Part model, mm, in its own coordinate system. A direction names the side the tool comes from. Round coordinates to 2 decimals unless told otherwise and drop trailing zeros. Loops run counter-clockwise (first coordinate to the right, second up) from the corner with the lowest first, then second, coordinate; pieces in that order, holes last.
1) Band-saw the part on C-C, the plane x = 53.5. Write the cut outline in (y, z), then the cut area to 3 significant figures.
2) Band-saw the part on D-D, the plane y = 48. Write the cut outline in (x, z).
3) 3-axis set-ups, long thin cutter, end or side, ignore diameter. For faces 1 (the flat face through (37, 38, 0)), 2 (the flat face through (37, 6.35, -42)): which of +Z, -Z, +X, -X, +Y, -Y reach the whole face in a straight line?
4) Band-saw the part on B-B, the plane x = 37.5. Write the cut outline in (y, z), then the cut area to 3 significant figures.
5) Band-saw the part on A-A, the plane z = -63.5. Write the cut outline in (x, y) (3 decimals), then the cut area to 3 significant figures.
6) Mould opens along Z. For faces 3 (the cylindrical face through (13.65, 3.13, -66.53)), 4 (the cylindrical face through (68.03, 23.45, -3.13)), 5 (the cylindrical face through (63.25, 3.13, -66.53)), 6 (the cylindrical face through (38.02, 7.85, -7.78)) say: +Z half, -Z half, draft (parallel to the pull), parting line (faces both ways), or undercut.
7) Probe line 1 (X direction, y = 4.5, z = -63.5) (3 decimals); line 2 (X direction, y = 60, z = -4); line 3 (Y direction, x = 69.5, z = -62). List the from-to ranges inside material, lowest first.
8) Drop flat-ended pins along their axis: P1, Ø5.5, axis at x = 62.3, z = -63.5, coming from the +Y side; P2, Ø1.5, axis at x = 14, z = -25.5, coming from the +Y side; P3, Ø14.5, axis at x = 37.5, y = 60, coming from the -Z side. Give the stop position or say it passes through.
from build123d import *

# Parameters (mm, degrees)
BOSS_EXTRUDE1_DEPTH = 75
FILLET1_R           = 3
FILLET2_R           = 5
SKETCH2_R           = 6.35
CUT_EXTRUDE1_DEPTH  = 132.293107207
SKETCH3_R           = 3.175
CUT_EXTRUDE2_DEPTH  = 132.293107207
SKETCH4_R           = 3.175
CUT_EXTRUDE3_DEPTH  = 132.293107207


with BuildPart() as part:
    # Sketch1 → Boss-Extrude1 (new body)
    with BuildSketch(Plane(origin=(0, 0, 0), x_dir=(0, 0, -1), z_dir=(1, 0, 0))):
        Polygon((0, 0), (0, 76.2), (6.35, 76.2), (6.35, 6.35), (76.2, 6.35), (76.2, 0), align=None)
    extrude(amount=BOSS_EXTRUDE1_DEPTH)

    # Fillet1
    fillet1_edges = [part.edges().sort_by_distance(p)[0] for p in [
        (37.5, 76.2, -6.35),
        (37.5, 6.35, -76.2),
    ]]
    fillet(fillet1_edges, radius=FILLET1_R)

    # Fillet2
    fillet2_edges = [part.edges().sort_by_distance(p)[0] for p in [
        (37.5, 6.35, -6.35),
    ]]
    fillet(fillet2_edges, radius=FILLET2_R)

    # Sketch2 → Cut-Extrude1 (cut, through all)
    with BuildSketch(Plane(origin=(0, 0, 0), x_dir=(-1, 0, 0), z_dir=(0, 0, -1))):
        with Locations(Location((-37.5, 60, 0), (0, 0, 180))):
            Circle(SKETCH2_R)
    extrude(amount=CUT_EXTRUDE1_DEPTH, mode=Mode.SUBTRACT)

    # Sketch3 → Cut-Extrude2 (cut, through all)
    with BuildSketch(Plane.XY):
        with Locations((10, 22.5)):
            Circle(SKETCH3_R)
        with Locations((65, 22.5)):
            Circle(SKETCH3_R)
    extrude(amount=-CUT_EXTRUDE2_DEPTH, mode=Mode.SUBTRACT)

    # Sketch4 → Cut-Extrude3 (cut, through all)
    with BuildSketch(Plane.XZ):
        with Locations(Location((12.7, -63.5, 0), (0, 0, 270))):
            Circle(SKETCH4_R)
        with Locations(Location((62.3, -63.5, 0), (0, 0, 270))):
            Circle(SKETCH4_R)
    extrude(amount=-CUT_EXTRUDE3_DEPTH, mode=Mode.SUBTRACT)


solid = part.part
Reported:
1. outline: (0, -76.2) - (3.35, -76.2) arc R3 ccw to (6.35, -73.2) - (6.35, -11.35) arc R5 cw to (11.35, -6.35) - (73.2, -6.35) arc R3 ccw to (76.2, -3.35) - (76.2, 0) - (0, 0) - close
1. area: 929 mm2
2. outline: (0, -6.35) - (75, -6.35) - (75, 0) - (0, 0) - close
3. face 1: +Z, +X, -X, +Y, -Y
3. face 2: -Z, +X, -X, +Y
4. outline: (0, -76.2) - (3.35, -76.2) arc R3 ccw to (6.35, -73.2) - (6.35, -11.35) arc R5 cw to (11.35, -6.35) - (53.65, -6.35) - (53.65, 0) - (0, 0) - close; (66.35, -6.35) - (73.2, -6.35) arc R3 ccw to (76.2, -3.35) - (76.2, 0) - (66.35, 0) - close
4. area: 848 mm2
5. outline: (0, 0) - (9.525, 0) - (9.525, 6.35) - (0, 6.35) - close; (15.875, 0) - (59.125, 0) - (59.125, 6.35) - (15.875, 6.35) - close; (65.475, 0) - (75, 0) - (75, 6.35) - (65.475, 6.35) - close
5. area: 396 mm2
6. face 3: undercut
6. face 4: draft
6. face 5: undercut
6. face 6: -Z half
7. line 1: x = 0 to 9.525, 15.875 to 59.125, 65.475 to 75
7. line 2: x = 0 to 31.15, 43.85 to 75
7. line 3: y = 0 to 6.35
8. P1: passes through
8. P2: stops at y = 6.35
8. P3: stops at z = -6.35
